Here's how the part is built. I have some questions about the finished solid (model axes, mm). Face numbers are marked on the shaded views. A direction names the side the tool comes from. Round coordinates to 2 decimals unless told otherwise and drop trailing zeros. Write each loop counter-clockwise with the first axis right and the second up, starting at its lowest first coordinate (ties: lowest second). Pieces come first, ordered by that corner, then holes. Notation, with made-up numbers: M 82,50 L 117,50 A26 cw 117,85 Z; hole C 20.5,45.5 d5. An arc over 180 degrees is marked long. Write item = value, one per line. Start each with the question number.
(1) I want a section at B-B (z = -18.75). List the corners of the cut face in (x, y) for me.
(2) I want a section at A-A (x = -12). List the corners of the cut face in (y, z) for me.
(3) I want a section at C-C (z = -3). List the corners of the cut face in (x, y) for me, and give its area (3 significant figures).
(4) Will these pins go through, and if not, where does the flat tip stop? pin 1 Ø3.5 at (x, z) = (-3, -27) entering from +Y; pin 2 Ø3 at (x, y) = (-12.5, 6.5) entering from +Z; pin 3 Ø5.5 at (x, z) = (-6, -3) entering from +Y.
(5) On a 3-axis mill with a long thin cutter (end or side, diameter ignored), from which of +Z, -Z, +X, -X, +Y, -Y can I reach the whole of each face in a straight line? I mean the marked faces 5, 6, 7, 8 and 9. Say none if no direction works.
(6) If we mould it in two halves opening along Y, with no side actions, what happens to the marked faces 1, 2, 3 and 4? For each: released by +Y, released by -Y, zero draft, split by the parting line, or undercut.
(7) I need wall thicknesses on line 1 along X through (y, z) = (2, -3); line 2 along Y through (x, z) = (-4.5, -14.25); line 3 along Z through (x, y) = (-14.25, 14). Which ranges of each line are inside material? Lowest first, please.
(8) I want a section at D-D (x = -1). List the corners of the cut face in (y, z) for me.
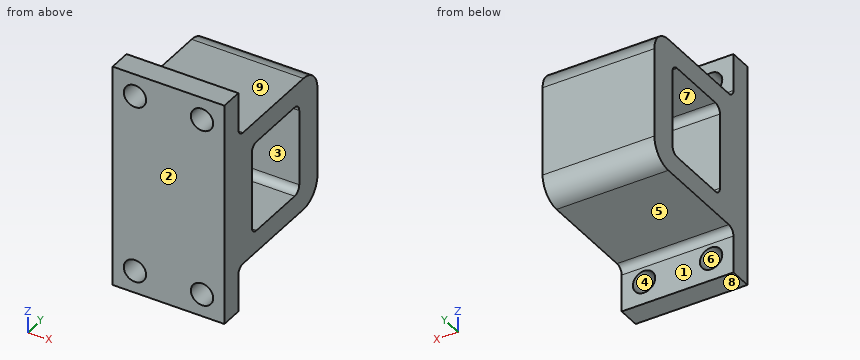
```python
from build123d import *

# Parameters (mm, degrees)
SKETCH1_W           = 15
SKETCH1_H           = 30
BOSS_EXTRUDE2_DEPTH = 3
SKETCH3_R           = 1.5
CUT_EXTRUDE1_DEPTH  = 3
SKETCH5_W           = 15
SKETCH5_H           = 9
BOSS_EXTRUDE3_DEPTH = 17
FILLET1_R           = 1
FILLET2_R           = 1
SKETCH6_W           = 12.2
SKETCH6_H           = 10.2
CUT_EXTRUDE2_DEPTH  = 40.05124838
FILLET3_R           = 3
FILLET4_R           = 3
FILLET5_R           = 1
FILLET6_R           = 1
FILLET7_R           = 1
FILLET8_R           = 1


with BuildPart() as part:
    # Sketch1 → Boss-Extrude2 (new body)
    with BuildSketch(Plane(origin=(0, 0, 0), x_dir=(1, 0, 0), z_dir=(0, 1, 0))):
        with Locations((-7.5, 15)):
            Rectangle(SKETCH1_W, SKETCH1_H)
    extrude(amount=BOSS_EXTRUDE2_DEPTH)

    # Sketch3 → Cut-Extrude1 (cut)
    with BuildSketch(Plane(origin=(0, 3, 0), x_dir=(1, 0, 0), z_dir=(0, 1, 0))):
        with Locations(Location((-12, 27, 0), (0, 0, 270))):
            Circle(SKETCH3_R)
        with Locations(Location((-3, 27, 0), (0, 0, 270))):
            Circle(SKETCH3_R)
        with Locations(Location((-3, 3, 0), (0, 0, 270))):
            Circle(SKETCH3_R)
        with Locations(Location((-12, 3, 0), (0, 0, 270))):
            Circle(SKETCH3_R)
    extrude(amount=-CUT_EXTRUDE1_DEPTH, mode=Mode.SUBTRACT)

    # Sketch5 → Boss-Extrude3 (add)
    with BuildSketch(Plane(origin=(0, 3, 0), x_dir=(1, 0, 0), z_dir=(0, 1, 0))):
        with Locations((-7.5, 19.5)):
            Rectangle(SKETCH5_W, SKETCH5_H)
        with Locations((-7.5, 10.5)):
            Rectangle(SKETCH5_W, SKETCH5_H)
    extrude(amount=BOSS_EXTRUDE3_DEPTH)

    # Fillet1
    fillet1_edges = [part.edges().sort_by_distance(p)[0] for p in [
        (-7.5, 3, -6),
    ]]
    fillet(fillet1_edges, radius=FILLET1_R)

    # Fillet2
    fillet2_edges = [part.edges().sort_by_distance(p)[0] for p in [
        (-7.5, 3, -24),
    ]]
    fillet(fillet2_edges, radius=FILLET2_R)

    # Sketch6 → Cut-Extrude2 (cut, through all)
    with BuildSketch(Plane(origin=(0, 0, 0), x_dir=(0, 0, -1), z_dir=(1, 0, 0))):
        with Locations((15, 11)):
            Rectangle(SKETCH6_W, SKETCH6_H)
    extrude(amount=-CUT_EXTRUDE2_DEPTH, mode=Mode.SUBTRACT)

    # Fillet3
    fillet3_edges = [part.edges().sort_by_distance(p)[0] for p in [
        (-7.5, 20, -24),
    ]]
    fillet(fillet3_edges, radius=FILLET3_R)

    # Fillet4
    fillet4_edges = [part.edges().sort_by_distance(p)[0] for p in [
        (-7.5, 20, -6),
    ]]
    fillet(fillet4_edges, radius=FILLET4_R)

    # Fillet5
    fillet5_edges = [part.edges().sort_by_distance(p)[0] for p in [
        (-7.5, 5.9, -8.9),
    ]]
    fillet(fillet5_edges, radius=FILLET5_R)

    # Fillet6
    fillet6_edges = [part.edges().sort_by_distance(p)[0] for p in [
        (-7.5, 16.1, -8.9),
    ]]
    fillet(fillet6_edges, radius=FILLET6_R)

    # Fillet7
    fillet7_edges = [part.edges().sort_by_distance(p)[0] for p in [
        (-7.5, 16.1, -21.1),
    ]]
    fillet(fillet7_edges, radius=FILLET7_R)

    # Fillet8
    fillet8_edges = [part.edges().sort_by_distance(p)[0] for p in [
        (-7.5, 5.9, -21.1),
    ]]
    fillet(fillet8_edges, radius=FILLET8_R)


solid = part.part
```
Returned:
q1.outline = M -15,0 L 0,0 L 0,5.9 L -15,5.9 Z; M -15,16.1 L 0,16.1 L 0,20 L -15,20 Z
q2.outline = M 0,-30 L 3,-30 L 3,-28.5 L 0,-28.5 Z; M 0,-25.5 L 3,-25.5 L 3,-25 A1 cw 4,-24 L 17,-24 A3 ccw 20,-21 L 20,-9 A3 ccw 17,-6 L 4,-6 A1 cw 3,-5 L 3,-4.5 L 0,-4.5 Z; M 0,-1.5 L 3,-1.5 L 3,0 L 0,0 Z; hole M 5.9,-20.1 A1 ccw 6.9,-21.1 L 15.1,-21.1 A1 ccw 16.1,-20.1 L 16.1,-9.9 A1 ccw 15.1,-8.9 L 6.9,-8.9 A1 ccw 5.9,-9.9 Z
q3.outline = M -15,0 L -13.5,0 L -13.5,3 L -15,3 Z; M -10.5,0 L -4.5,0 L -4.5,3 L -10.5,3 Z; M -1.5,0 L 0,0 L 0,3 L -1.5,3 Z
q3.area = 27.0 mm²
q4.pin_1 = 3
q4.pin_2 = -6
q4.pin_3 = 3.34
q5.face_5 = -Z, +X, -X, +Y
q5.face_6 = +Y, -Y
q5.face_7 = +X, -X
q5.face_8 = -Z, +X, -X, +Y, -Y
q5.face_9 = +Z, +X, -X, +Y
q6.face_1 = released by +Y
q6.face_2 = released by -Y
q6.face_3 = undercut
q6.face_4 = zero draft
q7.line_1 = -15 to -13.5, -10.5 to -4.5, -1.5 to 0
q7.line_2 = 0 to 5.9, 16.1 to 20
q7.line_3 = -24 to -21.1, -8.9 to -6
q8.outline = M 0,-30 L 3,-30 L 3,-25 A1 cw 4,-24 L 17,-24 A3 ccw 20,-21 L 20,-9 A3 ccw 17,-6 L 4,-6 A1 cw 3,-5 L 3,0 L 0,0 Z; hole M 5.9,-20.1 A1 ccw 6.9,-21.1 L 15.1,-21.1 A1 ccw 16.1,-20.1 L 16.1,-9.9 A1 ccw 15.1,-8.9 L 6.9,-8.9 A1 ccw 5.9,-9.9 Z
